```python
from build123d import *

# Parameters (mm, degrees)
BOSS_EXTRUDE1_DEPTH   = 4.7625
F_6_CLEARANCE_HOLE1_D = 4.3053
SKETCH6_R             = 9.525
CUT_EXTRUDE1_DEPTH    = 5.7625


with BuildPart() as part:
    # Sketch1 → Boss-Extrude1 (new body)
    with BuildSketch(Plane.XY):
        with BuildLine():
            Line((61.328308874, -51.443881834), (72.233641051, -46.509447198))
            ThreePointArc((72.233641051, -46.509447198), (73.031430575, -45.658526875), (72.993861427, -44.492712962))
            Line((72.993861427, -44.492712962), (23.309209228, 65.312700679))
            ThreePointArc((23.309209228, 65.312700679), (22.458288905, 66.110490204), (21.292474992, 66.072921056))
            Line((21.292474992, 66.072921056), (10.387142815, 61.13848642))
            ThreePointArc((10.387142815, 61.13848642), (5.529584843, 60.981948303), (1.984083498, 64.306071322))
            Line((1.984083498, 64.306071322), (0.923899929, 66.649126776))
            ThreePointArc((0.923899929, 66.649126776), (0.072979606, 67.4469163), (-1.092834307, 67.409347153))
            Line((-1.092834307, 67.409347153), (-38.813134462, 50.341700559))
            ThreePointArc((-38.813134462, 50.341700559), (-39.610923987, 49.490780236), (-39.573354839, 48.324966323))
            Line((-39.573354839, 48.324966323), (-38.51317127, 45.981910869))
            ThreePointArc((-38.51317127, 45.981910869), (-38.356633153, 41.124352897), (-41.680756172, 37.578851552))
            Line((-41.680756172, 37.578851552), (-52.586088348, 32.644416915))
            ThreePointArc((-52.586088348, 32.644416915), (-53.383877873, 31.793496593), (-53.346308725, 30.627682679))
            Line((-53.346308725, 30.627682679), (-3.661656526, -79.177730962))
            ThreePointArc((-3.661656526, -79.177730962), (-2.810736203, -79.975520486), (-1.64492229, -79.937951338))
            Line((-1.64492229, -79.937951338), (9.260409887, -75.003516702))
            ThreePointArc((9.260409887, -75.003516702), (14.117967859, -74.846978586), (17.663469204, -78.171101604))
            Line((17.663469204, -78.171101604), (18.723652773, -80.514157058))
            ThreePointArc((18.723652773, -80.514157058), (19.574573096, -81.311946583), (20.740387009, -81.274377435))
            Line((20.740387009, -81.274377435), (58.460687164, -64.206730842))
            ThreePointArc((58.460687164, -64.206730842), (59.258476689, -63.355810519), (59.220907541, -62.189996606))
            Line((59.220907541, -62.189996606), (58.160723972, -59.846941151))
            ThreePointArc((58.160723972, -59.846941151), (58.004185856, -54.989383179), (61.328308874, -51.443881834))
        make_face()
    extrude(amount=BOSS_EXTRUDE1_DEPTH)

    # #6 Clearance Hole1 (through all)
    with Locations(Plane.XY.offset(4.7625)):
        with Locations((30.114722566, 23.855073088), (46.082919532, -11.435391781), (-33.128884005, 16.984419854), (21.298547528, -42.304619004)):
            Hole(F_6_CLEARANCE_HOLE1_D / 2)

    # Sketch6 → Cut-Extrude1 (cut, through all)
    with BuildSketch(Plane.XY.offset(4.7625)):
        with Locations((13.026989476, 37.590195142)):
            Circle(SKETCH6_R)
        with Locations((28.942831698, 2.415436715)):
            Circle(SKETCH6_R)
        with Locations((44.858673919, -32.759321712)):
            Circle(SKETCH6_R)
        with Locations((-16.503976684, 3.039878823)):
            Circle(SKETCH6_R)
        with Locations((-0.588134462, -32.134879603)):
            Circle(SKETCH6_R)
        with Locations((-29.802081698, 32.42931514)):
            Circle(SKETCH6_R)
        with Locations((12.395842088, -60.830077267)):
            Circle(SKETCH6_R)
    extrude(amount=-CUT_EXTRUDE1_DEPTH, mode=Mode.SUBTRACT)


solid = part.part
```
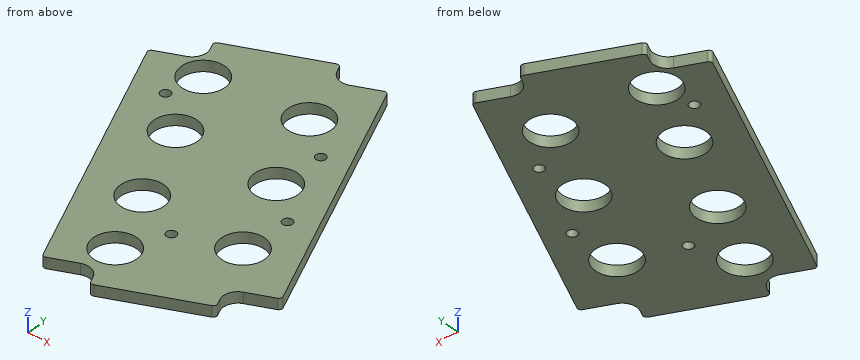
Can you work these out from the model? Positions are in its coordinate system, mm. Round coordinates to 2 decimals unless told otherwise and drop trailing zeros. Loops run counter-clockwise (first coordinate to the right, second up) from the corner with the lowest first, then second, coordinate; pieces in that order, holes last. Notation, with made-up numbers: (34.25, -2) -> (38.25, -2) arc R15 cw to (38.25, 23) -> close; hole circle Ø3 at (61, 33.5). An arc over 180 degrees is marked (long way). Answer in a Markdown table with one row per item.
Item 1: Will these pins go through, and if not, where does the flat tip stop? P1, Ø2, axis at y = 11, z = 1.5, coming from the +X side; P2, Ø15, axis at x = -29.8, y = 32.43, coming from the +Z side; P3, Ø1, axis at x = 17.5, z = 3, coming from the -Y side; P4, Ø1.5, axis at y = -27, z = 4, coming from the -X side.
Answer block:
| item | result |
|---|---|
| P1 | x = 48.34 |
| P2 | through |
| P3 | y = -78.91 |
| P4 | x = -27.61 |
Item 2: Suppose I cut it at A-A, the plane y = 10. List the corners of the cut face in (x, z) for me.
Answer block:
| item | result |
|---|---|
| outline | (-44.01, 0) -> (-23.01, 0) -> (-23.01, 4.76) -> (-44.01, 4.76) -> close; (-10, 0) -> (23.18, 0) -> (23.18, 4.76) -> (-10, 4.76) -> close; (34.7, 0) -> (48.34, 0) -> (48.34, 4.76) -> (34.7, 4.76) -> close |
Item 3: Suppose I cut it at C-C, the plane y = -68. List the corners of the cut face in (x, z) for me.
Answer block:
| item | result |
|---|---|
| outline | (-8.72, 0) -> (6.13, 0) -> (6.13, 4.76) -> (-8.72, 4.76) -> close; (18.67, 0) -> (50.08, 0) -> (50.08, 4.76) -> (18.67, 4.76) -> close |
Item 4: If I drill on probe 1 along X at (y, z) = (-3, 3.95); probe 2 along Y at (x, z) = (-34, 1.8); probe 3 along Y at (x, z) = (-33, 1.3), over which ranges is the centre line in solid material (lowest first)?
Answer block:
| item | result |
|---|---|
| probe 1 | -38.13 to -23.87, -9.14 to 21.11, 36.78 to 54.22 |
| probe 2 | -12.13 to 15.02, 18.95 to 23.88, 40.98 to 52.52 |
| probe 3 | -14.34 to 14.84, 19.13 to 23.46, 41.4 to 52.97 |
Item 5: Suppose I cut it at D-D, the plane z = 1.85. Give the number of separate pieces and of enclosed holes in the cut face, plus the area to 3 significant figures.
Answer block:
| item | result |
|---|---|
| separate pieces | 1 |
| enclosed holes | 11 |
| area | 9,300 mm² |
Item 6: Suppose I cut it at B-B, the plane x = -33. List the corners of the cut face in (y, z) for me.
Answer block:
| item | result |
|---|---|
| outline | (-14.34, 0) -> (14.84, 0) -> (14.84, 4.76) -> (-14.34, 4.76) -> close; (19.13, 0) -> (23.46, 0) -> (23.46, 4.76) -> (19.13, 4.76) -> close; (41.4, 0) -> (52.97, 0) -> (52.97, 4.76) -> (41.4, 4.76) -> close |
